Model file for the job. Use its own axes, mm. Face numbers are marked on the shaded views. A direction names the side the tool comes from. Coordinates: 2 decimals unless noted, no trailing zeros. Write each loop counter-clockwise with the first axis right and the second up, starting at its lowest first coordinate (ties: lowest second). Pieces come first, ordered by that corner, then holes. Notation, with made-up numbers: (86.25, 53) - (99.25, 53) arc R21 cw to (99.25, 83) - close; hole circle Ø4 at (63.25, -5.5). An arc over 180 degrees is marked (long way). Put each result on its own line as item: value. Start each with the question number.
1. Saw through at D-D, the plane x = 8. Write the cut outline in (y, z).
2. Drop flat-ended pins along their axis: P1, Ø0.8, axis at x = 4, y = -8.5, coming from the +Z side; P2, Ø8, axis at x = -1, z = 13.5, coming from the +Y side; P3, Ø5, axis at x = -3.5, z = 5.5, coming from the -Y side. Give the stop position or say it passes through.
3. Saw through at C-C, the plane y = 0. Write the cut outline in (x, z).
4. Saw through at B-B, the plane z = 9. Write the cut outline in (x, y), plus the area to 3 significant figures.
5. Which spindle directions (+Z, -Z, +X, -X, +Y, -Y) get a long thin tool onto all of the face, cutting with end or side? Do the marked faces 1, 2, 3, 4 and 5. Say none if no direction does.
6. Drill centre lines: L1, parallel to Y at x = -5, z = 9; L2, parallel to Z at x = -2, y = 0; L3, parallel to Z at x = 6.5, y = 5.5. Where is each one in solid material? Low to high. Write a range as from..to.
7. Saw through at A-A, the plane x = 0. Write the cut outline in (y, z).
```python
from build123d import *

# Parameters (mm, degrees)
F0_W          = 19
F0_H          = 19
F3_DEPTH      = 2
F4_START      = 2
F2_W          = 19
F2_H          = 14
F4_DEPTH      = 9.5
F5_START      = 11.5
F1_R          = 6
F5_DEPTH      = 7.5
F6_R          = 1
F7_DEPTH      = 25
F7_DEPTH_BACK = 25


with BuildPart() as f3:
    # F0 (on Top) → F3 (new body)
    with BuildSketch(Plane.XY):
        Rectangle(F0_W, F0_H)
    extrude(amount=F3_DEPTH)

    # F2 (on Top) → F4 (join)
    with BuildSketch(Plane.XY.offset(F4_START)):
        Rectangle(F2_W, F2_H)
    extrude(amount=F4_DEPTH)

    # F1 (on Top) → F5 (join)
    with BuildSketch(Plane.XY.offset(F5_START)):
        Circle(F1_R)
    extrude(amount=F5_DEPTH)

    # F6 (on Right) → F7 (cut, two sides)
    with BuildSketch(Plane.YZ) as f7_sk:
        with Locations((0, 9)):
            Circle(F6_R)
    extrude(amount=-F7_DEPTH, mode=Mode.SUBTRACT)
    extrude(f7_sk.sketch, amount=F7_DEPTH_BACK, mode=Mode.SUBTRACT)


solid = f3.part
```
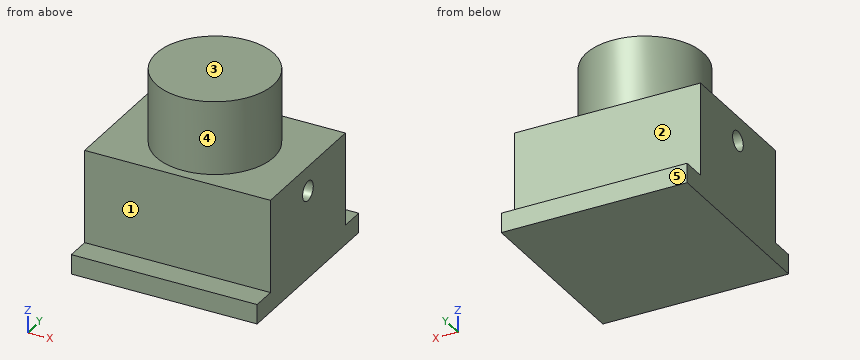
Final values:
1. outline: (-9.5, 0) - (9.5, 0) - (9.5, 2) - (7, 2) - (7, 11.5) - (-7, 11.5) - (-7, 2) - (-9.5, 2) - close; hole circle Ø2 at (0, 9)
2. P1: stops at z = 2
2. P2: stops at y = 7
2. P3: stops at y = -7
3. outline: (-9.5, 0) - (9.5, 0) - (9.5, 8) - (-9.5, 8) - close; (-9.5, 10) - (9.5, 10) - (9.5, 11.5) - (6, 11.5) - (6, 19) - (-6, 19) - (-6, 11.5) - (-9.5, 11.5) - close
4. outline: (-9.5, -7) - (9.5, -7) - (9.5, -1) - (-9.5, -1) - close; (-9.5, 1) - (9.5, 1) - (9.5, 7) - (-9.5, 7) - close
4. area: 228 mm²
5. face 1: +Z, +X, -X, -Y
5. face 2: +Z, +X, -X, +Y
5. face 3: +Z, +X, -X, +Y, -Y
5. face 4: +Z
5. face 5: +Z, -Z, +X, -X, +Y
6. L1: y = -7..-1, 1..7
6. L2: z = 0..8, 10..19
6. L3: z = 0..11.5
7. outline: (-9.5, 0) - (9.5, 0) - (9.5, 2) - (7, 2) - (7, 11.5) - (6, 11.5) - (6, 19) - (-6, 19) - (-6, 11.5) - (-7, 11.5) - (-7, 2) - (-9.5, 2) - close; hole circle Ø2 at (0, 9)
